For this review, take the finished solid that the model builds, in its own axes (mm). Give positions to 0.01 mm unless a question says otherwise; leave off trailing zeros. Order: outer loops, then holes, each group sorted by start corner. A loop starts at its lowest first (then second) coordinate and runs counter-clockwise, first axis right, second up.
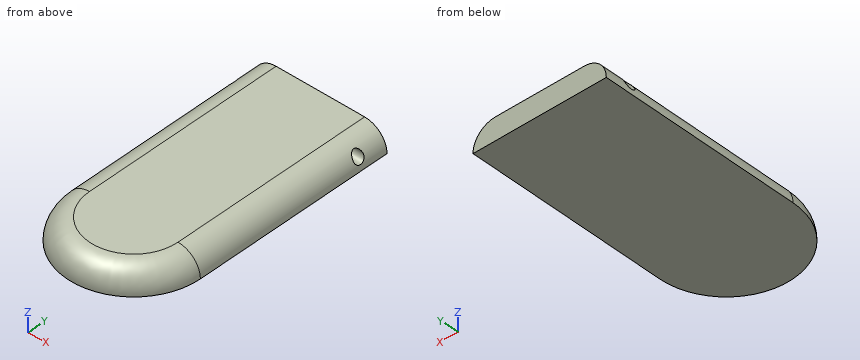
from build123d import *

# Parameters (mm, degrees)
EXTRUDE_1_DEPTH     = 10
SKETCH_9_R          = 2.5
CUT_EXTRUDE_1_DEPTH = 59.5
FILLET_3_R          = 10


with BuildPart() as part:
    # Эскиз1 → Бобышка-Вытянуть1 (new body)
    with BuildSketch(Plane.XY):
        with BuildLine():
            Line((0, 0), (59.5, 0))
            Line((59.5, 0), (59.5, -90.25))
            ThreePointArc((59.5, -90.25), (29.75, -120), (0, -90.25))
            Line((0, -90.25), (0, 0))
        make_face()
    extrude(amount=EXTRUDE_1_DEPTH)

    # Эскиз9 → Вырез-Вытянуть1 (cut)
    with BuildSketch(Plane(origin=(59.5, 0, 0), x_dir=(0, 0, -1), z_dir=(1, 0, 0))):
        with Locations(Location((-5, -12.5, 0), (0, 0, 90))):
            Circle(SKETCH_9_R)
    extrude(amount=-CUT_EXTRUDE_1_DEPTH, mode=Mode.SUBTRACT)

    # Скругление3
    # the kernel refuses this fillet: 10 mm, written as the material it takes off along each edge
    with BuildSketch(Plane(origin=(0, -90.25, 10), x_dir=(0, 0, -1), z_dir=(0, 1, 0)), Plane(origin=(59.5, 25, 10), x_dir=(0, 0, -1), z_dir=(0, -1, 0))) as fillet_3_piece_1:
        with BuildLine():
            CenterArc((FILLET_3_R, -FILLET_3_R), FILLET_3_R, 90, 90)
            Line((0, -FILLET_3_R), (0, 0))
            Line((0, 0), (FILLET_3_R, 0))
        make_face()
    extrude(amount=115.25, mode=Mode.SUBTRACT)
    with BuildSketch(Plane(origin=(29.75, -90.25, 10), x_dir=(1, 0, 0), z_dir=(0, 1, 0))) as fillet_3_piece_2:
        with BuildLine():
            CenterArc((29.75 - FILLET_3_R, FILLET_3_R), FILLET_3_R, 270, 90)
            Line((29.75 - FILLET_3_R, 0), (29.75, 0))
            Line((29.75, 0), (29.75, FILLET_3_R))
        make_face()
    revolve(axis=Axis((29.75, -90.25, 10), (0, 0, -1)), revolution_arc=180, mode=Mode.SUBTRACT)


solid = part.part
1) We need section C-C on y = -54. Give the boundary of the cut face in (x, z).
Answer sheet:
outline: (0, 0) - (59.5, 0) arc R10 ccw to (49.5, 10) - (10, 10) arc R10 ccw to start
2) We need section B-B on y = -13.5. Give the boundary of the cut face in (x, z).
Answer sheet:
outline: (0, 0) - (59.5, 0) arc R10 ccw to (59.13, 2.71) - (0.37, 2.71) arc R10 ccw to start; (3.16, 7.29) - (56.34, 7.29) arc R10 ccw to (49.5, 10) - (10, 10) arc R10 ccw to start
3) To check wall thickness, follow line 1 (Z direction, x = 25, y = -12.5); line 2 (X direction, y = -45, z = 2.5); line 3 (Y direction, x = 42, z = 5). State the ranges of each line that lie inside material, in increasing order.
Answer sheet:
line 1: z = 0 to 2.5, 7.5 to 10
line 2: x = 0.32 to 59.18
line 3: y = -115.88 to -15, -10 to 0
4) Clearance check with flat-ended pins moving along their axes: pin 1 (5 mm diameter, centred on x = 34.5, z = 4.5, fed in from -Y); pin 2 (3 mm diameter, centred on y = -12.5, z = 5, fed in from +X). State where each tip first meets the part, or that it passes through.
Answer sheet:
pin 1: stops at y = -119.52
pin 2: passes through
5) We need section A-A on z = 6.25. Give the boundary of the cut face in (x, y), then the cut area to 3 significant figures.
Answer sheet:
outline: (2.19, -90.25) arc R27.56 ccw to (57.31, -90.25) - (57.31, -14.67) - (2.19, -14.67) - close; (2.19, -10.33) - (57.31, -10.33) - (57.31, 0) - (2.19, 0) - close
area: 5,930 mm2
